from build123d import *

# Parameters (mm, degrees)
SKETCH1_W           = 25.4
SKETCH1_H           = 57.15
BOSS_EXTRUDE1_DEPTH = 1.5875
SKETCH2_R           = 1.5875
CUT_EXTRUDE2_DEPTH  = 2.5875
FILLET1_R           = 3.175


with BuildPart() as part:
    # Sketch1 → Boss-Extrude1 (new body)
    with BuildSketch(Plane(origin=(0, 0, 0), x_dir=(1, 0, 0), z_dir=(0, 1, 0))):
        with Locations((12.7, 28.575)):
            Rectangle(SKETCH1_W, SKETCH1_H)
    extrude(amount=BOSS_EXTRUDE1_DEPTH)

    # Sketch2 → Cut-Extrude2 (cut, through all)
    with BuildSketch(Plane(origin=(0, 1.5875, 0), x_dir=(1, 0, 0), z_dir=(0, 1, 0))):
        with Locations((2.38125, 54.76875)):
            Circle(SKETCH2_R)
        with Locations((23.01875, 54.76875)):
            Circle(SKETCH2_R)
        with Locations((23.01875, 2.38125)):
            Circle(SKETCH2_R)
        with Locations((2.38125, 2.38125)):
            Circle(SKETCH2_R)
    extrude(amount=-CUT_EXTRUDE2_DEPTH, mode=Mode.SUBTRACT)

    # Fillet1
    fillet1_edges = [part.edges().sort_by_distance(p)[0] for p in [
        (0, 0.79375, -57.15),
        (25.4, 0.79375, -57.15),
        (25.4, 0.79375, 0),
        (0, 0.79375, 0),
    ]]
    fillet(fillet1_edges, radius=FILLET1_R)


solid = part.part
The listing builds one solid part. Answer for the finished solid, in the listing's coordinates (mm). Coordinates: 2 decimals unless noted, no trailing zeros. Order: outer loops, then holes, each group sorted by start corner. A loop starts at its lowest first (then second) coordinate and runs counter-clockwise, first axis right, second up.
Q1. A cutting plane is placed at A-A, the plane x = 23.25. Write down the section's boundary in (y, z), and give its area (3 significant figures).
Q2. A cutting plane is placed at B-B, the plane y = 1.2. State how many separate pieces and enclosed holes the cut face has, and give its area (3 significant figures).
Q3. For a pull along X with two mould halves and no side action, classify faces 1 (the face through (22.67, 0.8, -53.22)), 2 (the face through (3.848, 0.805, -1.773)), 3 (the face through (25.4, 1, -28)), 4 (the face through (13, 1, -57.15)) as pulls with the +X half, pulls with the -X half, needs draft (parallel to the pull), parting line crosses it, or undercut.
Q4. Given P1, Ø3, axis at x = 2.38, z = -2.38, coming from the -Y side, flat-ended and moving along its own axis, determine where the tip first touches the part or whether it passes through.
Q5. Consider line 1 (Z direction, x = 2.75, y = 0.65); line 2 (Z direction, x = 3.5, y = 0.75). Determine where each line is inside the solid, lowest interval first.
Answers follow:
1. outline: (0, -56.98) - (1.59, -56.98) - (1.59, -56.34) - (0, -56.34) - close; (0, -53.2) - (1.59, -53.2) - (1.59, -3.95) - (0, -3.95) - close; (0, -0.81) - (1.59, -0.81) - (1.59, -0.17) - (0, -0.17) - close
1. area: 80.2 mm2
2. separate pieces: 1
2. enclosed holes: 4
2. area: 1,410 mm2
3. face 1: undercut
3. face 2: undercut
3. face 3: pulls with the +X half
3. face 4: needs draft
4. P1: passes through
5. line 1: z = -57.12 to -56.31, -53.22 to -3.93, -0.84 to -0.03
5. line 2: z = -57.15 to -55.9, -53.64 to -3.51, -1.25 to 0
